```python
from build123d import *

# Parameters (mm, degrees)
F0_W     = 914.4
F0_H     = 323.85
F1_DEPTH = 82.55
F2_W     = 876.3
F2_H     = 285.75
F3_DEPTH = 82.55
F4_W     = 19.05
F4_H     = 285.75
F5_DEPTH = 82.55
F6_W     = 19.05
F6_H     = 285.75
F7_DEPTH = 82.55
F8_W     = 19.05
F8_H     = 285.75
F9_DEPTH = 82.55


with BuildPart() as f1:
    # F0 (on Top) → F1 (new body)
    with BuildSketch(Plane.XY):
        Rectangle(F0_W, F0_H)
    extrude(amount=F1_DEPTH)

    # F2 (on face) → F3 (cut)
    with BuildSketch(Plane(origin=(0, 0, 0), x_dir=(1, 0, 0), z_dir=(0, 0, -1))):
        Rectangle(F2_W, F2_H)
    extrude(amount=-F3_DEPTH, mode=Mode.SUBTRACT)

    # F4 (on face) → F5 (join)
    with BuildSketch(Plane(origin=(0, 0, 0), x_dir=(1, 0, 0), z_dir=(0, 0, -1))):
        Rectangle(F4_W, F4_H)
    extrude(amount=-F5_DEPTH)

    # F6 (on face) → F7 (join)
    with BuildSketch(Plane(origin=(0, 0, 0), x_dir=(1, 0, 0), z_dir=(0, 0, -1))):
        with Locations((-223.8375, 0)):
            Rectangle(F6_W, F6_H)
    extrude(amount=-F7_DEPTH)

    # F8 (on face) → F9 (join)
    with BuildSketch(Plane(origin=(0, 0, 0), x_dir=(1, 0, 0), z_dir=(0, 0, -1))):
        with Locations((223.8375, 0)):
            Rectangle(F8_W, F8_H)
    extrude(amount=-F9_DEPTH)


solid = f1.part
```
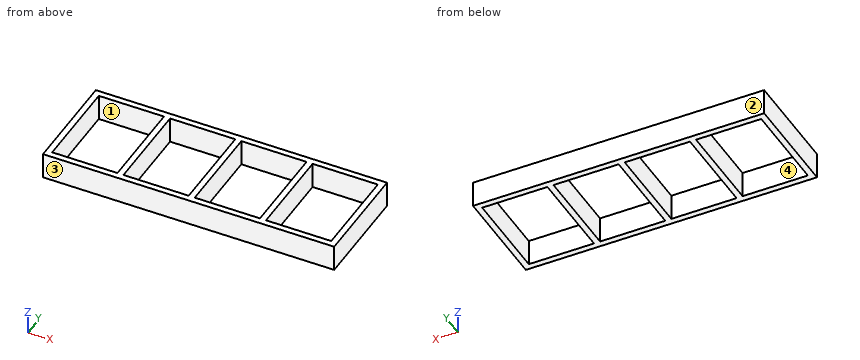
Geometry: final body of the model. Coordinates: model frame, mm. Face numbers are marked on the shaded views. A direction names the side the tool comes from. Coordinates: 2 decimals unless noted, no trailing zeros. Order: outer loops, then holes, each group sorted by start corner. A loop starts at its lowest first (then second) coordinate and runs counter-clockwise, first axis right, second up. Notation, with made-up numbers: (18.25, 14.5) -> (27.25, 14.5) arc R23 ccw to (27.25, 24.5) -> close; hole circle Ø6 at (-27, -18). An arc over 180 degrees is marked (long way). Use CSV: the item, a comma, the result in double quotes.
1) Section C-C on x = -22.5. Output: boundary loops of the cut face in (y, z) (3 decimals), then the cut area to 3 significant figures.
Findings:
outline,"(-161.925, 0) -> (-142.875, 0) -> (-142.875, 82.55) -> (-161.925, 82.55) -> close; (142.875, 0) -> (161.925, 0) -> (161.925, 82.55) -> (142.875, 82.55) -> close"
area,"3,150 mm^2"
2) Mould query, pull axis X, two halves, no side actions, for the marked faces 1 and 2. Classes: +X half, -X half, draft (parallel to the pull), parting line (faces both ways), or undercut.
Findings:
face 1,"undercut"
face 2,"draft"
3) Line query: line 1 (Y direction, x = 296, z = 36) (3 decimals). Output: solid intervals per line, ascending.
Findings:
line 1,"y = -161.925 to -142.875, 142.875 to 161.925"
4) Section A-A on z = 49. State how many separate pieces and enclosed holes the cut face has, then the cut area to 3 significant figures.
Findings:
separate pieces,"1"
enclosed holes,"4"
area,"62,100 mm^2"
5) Access query for the marked faces 3 and 4. Directions: +Z, -Z, +X, -X, +Y, -Y. A direction counts if a zero-diameter tool reaches every point of the face in a straight line with its end or side. Return the directions, or none.
Findings:
face 3,"+Z, -Z, +X, -X, -Y"
face 4,"+Z, -Z"
